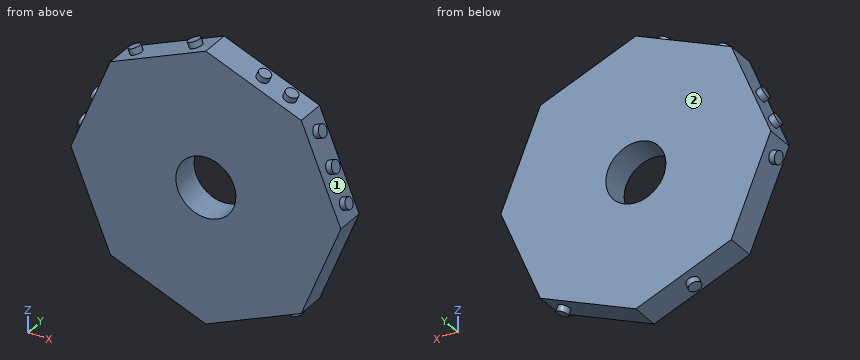
from build123d import *

# Parameters (mm, degrees)
BOSS_EXTRUDE1_DEPTH      = 12.7
SKETCH6_R                = 2.582336278
BOSS_EXTRUDE5_DEPTH      = 2.54
SKETCH8_R                = 2.650649738
BOSS_EXTRUDE7_DEPTH      = 2.54
SKETCH9_R                = 2.655151376
BOSS_EXTRUDE8_DEPTH      = 2.54
BOSS_EXTRUDE9_DEPTH      = 2.54
BOSS_EXTRUDE9_DEPTH_BACK = 2.032
SKETCH10_R               = 2.513561162
SKETCH11_R               = 2.58621177
BOSS_EXTRUDE10_DEPTH     = 2.54
SKETCH12_R               = 2.635427952
BOSS_EXTRUDE11_DEPTH     = 2.54
SKETCH13_R               = 2.610060734
BOSS_EXTRUDE12_DEPTH     = 2.54
SKETCH14_R               = 2.635257061
BOSS_EXTRUDE13_DEPTH     = 2.54
SKETCH15_R               = 2.496375984
BOSS_EXTRUDE14_DEPTH     = 2.54
SKETCH16_R               = 2.621965254
BOSS_EXTRUDE15_DEPTH     = 2.54
SKETCH17_R               = 2.649584499
BOSS_EXTRUDE16_DEPTH     = 2.54
SKETCH18_R               = 2.417668351
BOSS_EXTRUDE17_DEPTH     = 2.54
SKETCH25_R               = 12.696845274
CUT_EXTRUDE1_DEPTH       = 12.954


with BuildPart() as part:
    # Sketch2 → Boss-Extrude1 (new body)
    with BuildSketch(Plane(origin=(0, 0, 0), x_dir=(1, 0, 0), z_dir=(0, 1, 0))):
        Polygon((57.113851186, 0), (40.385591473, 40.385591473), (0, 57.113851186), (-40.385591473, 40.385591473), (-57.113851186, 0), (-40.385591473, -40.385591473), (0, -57.113851186), (40.385591473, -40.385591473), align=None)
    extrude(amount=BOSS_EXTRUDE1_DEPTH)

    # Sketch6 → Boss-Extrude5 (add)
    with BuildSketch(Plane(origin=(20.192795737, 0, 48.749721329), x_dir=(0.9238795325112822, 0, -0.38268343236510083), z_dir=(0.38268343236510083, 0, 0.9238795325112822))):
        with Locations(Location((0, 6.35, 0), (0, 0, 180))):
            Circle(SKETCH6_R)
    extrude(amount=BOSS_EXTRUDE5_DEPTH)

    # Sketch8 → Boss-Extrude7 (add)
    with BuildSketch(Plane(origin=(20.192795737, 0, 48.749721329), x_dir=(0.9238795325112822, 0, -0.38268343236510083), z_dir=(0.38268343236510083, 0, 0.9238795325112822))):
        with Locations(Location((12.369517224, 6.35, 0), (0, 0, 180))):
            Circle(SKETCH8_R)
    extrude(amount=BOSS_EXTRUDE7_DEPTH)

    # Sketch9 → Boss-Extrude8 (add)
    with BuildSketch(Plane(origin=(-20.192795737, 0, 48.749721329), x_dir=(0.9238795325112911, 0, 0.38268343236507935), z_dir=(-0.38268343236507935, 0, 0.9238795325112911))):
        with Locations(Location((13.282722146, 6.35, 0), (0, 0, 180))):
            Circle(SKETCH9_R)
    extrude(amount=BOSS_EXTRUDE8_DEPTH)

    # Sketch10 → Boss-Extrude9 (add, two sides: drawn at the far end of the back side and taken through both)
    with BuildSketch(Plane(origin=(-20.192795737, 0, 48.749721329), x_dir=(0.9238795325112911, 0, 0.38268343236507935), z_dir=(-0.38268343236507935, 0, 0.9238795325112911)).offset(-BOSS_EXTRUDE9_DEPTH_BACK)):
        with Locations(Location((-14.008863044, 6.35, 0), (0, 0, 180))):
            Circle(SKETCH10_R)
    extrude(amount=BOSS_EXTRUDE9_DEPTH + BOSS_EXTRUDE9_DEPTH_BACK)

    # Sketch11 → Boss-Extrude10 (add)
    with BuildSketch(Plane(origin=(-48.749721329, 0, 20.192795737), x_dir=(0.3826834323651003, 0, 0.9238795325112825), z_dir=(-0.9238795325112825, 0, 0.3826834323651003))):
        with Locations(Location((-13.637069306, 6.35, 0), (0, 0, 180))):
            Circle(SKETCH11_R)
    extrude(amount=BOSS_EXTRUDE10_DEPTH)

    # Sketch12 → Boss-Extrude11 (add)
    with BuildSketch(Plane(origin=(-48.749721329, 0, 20.192795737), x_dir=(0.3826834323651003, 0, 0.9238795325112825), z_dir=(-0.9238795325112825, 0, 0.3826834323651003))):
        with Locations(Location((0, 6.35, 0), (0, 0, 180))):
            Circle(SKETCH12_R)
    extrude(amount=BOSS_EXTRUDE11_DEPTH)

    # Sketch13 → Boss-Extrude12 (add)
    with BuildSketch(Plane(origin=(-48.749721329, 0, -20.192795737), x_dir=(-0.38268343236507907, 0, 0.9238795325112913), z_dir=(-0.9238795325112913, 0, -0.38268343236507907))):
        with Locations(Location((14.354264816, 6.35, 0), (0, 0, 180))):
            Circle(SKETCH13_R)
    extrude(amount=BOSS_EXTRUDE12_DEPTH)

    # Sketch14 → Boss-Extrude13 (add)
    with BuildSketch(Plane(origin=(-20.192795737, 0, -48.749721329), x_dir=(-0.9238795325112825, 0, 0.3826834323651002), z_dir=(-0.3826834323651002, 0, -0.9238795325112825))):
        with Locations(Location((0, 6.35, 0), (0, 0, 180))):
            Circle(SKETCH14_R)
    extrude(amount=BOSS_EXTRUDE13_DEPTH)

    # Sketch15 → Boss-Extrude14 (add)
    with BuildSketch(Plane(origin=(20.192795737, 0, -48.749721329), x_dir=(-0.9238795325112913, 0, -0.38268343236507896), z_dir=(0.3826834323650789, 0, -0.9238795325112912))):
        with Locations(Location((-15.021400656, 6.35, 0), (0, 0, 180))):
            Circle(SKETCH15_R)
    extrude(amount=BOSS_EXTRUDE14_DEPTH)

    # Sketch16 → Boss-Extrude15 (add)
    with BuildSketch(Plane(origin=(48.749721329, 0, 20.192795737), x_dir=(0.3826834323650791, 0, -0.9238795325112912), z_dir=(0.9238795325112913, 0, 0.3826834323650792))):
        with Locations(Location((-14.377366693, 6.35, 0), (0, 0, 180))):
            Circle(SKETCH16_R)
    extrude(amount=BOSS_EXTRUDE15_DEPTH)

    # Sketch17 → Boss-Extrude16 (add)
    with BuildSketch(Plane(origin=(48.749721329, 0, 20.192795737), x_dir=(0.3826834323650791, 0, -0.9238795325112912), z_dir=(0.9238795325112913, 0, 0.3826834323650792))):
        with Locations(Location((0, 6.35, 0), (0, 0, 180))):
            Circle(SKETCH17_R)
    extrude(amount=BOSS_EXTRUDE16_DEPTH)

    # Sketch18 → Boss-Extrude17 (add)
    with BuildSketch(Plane(origin=(48.749721329, 0, 20.192795737), x_dir=(0.3826834323650791, 0, -0.9238795325112912), z_dir=(0.9238795325112913, 0, 0.3826834323650792))):
        with Locations(Location((14.696818613, 6.35, 0), (0, 0, 180))):
            Circle(SKETCH18_R)
    extrude(amount=BOSS_EXTRUDE17_DEPTH)

    # Sketch25 → Cut-Extrude1 (cut)
    with BuildSketch(Plane(origin=(0, 12.7, 0), x_dir=(1, 0, 0), z_dir=(0, 1, 0))):
        with Locations(Location((0, 0, 0), (0, 0, 270))):
            Circle(SKETCH25_R)
    extrude(amount=-CUT_EXTRUDE1_DEPTH, mode=Mode.SUBTRACT)


solid = part.part
CAD build for the part. Positions are in the model's coordinates, mm. Face numbers are marked on the shaded views. Round coordinates to 2 decimals unless told otherwise and drop trailing zeros. Order: outer loops, then holes, each group sorted by start corner. A loop starts at its lowest first (then second) coordinate and runs counter-clockwise, first axis right, second up. Notation, with made-up numbers: (62.5, 88.5) - (88.5, 88.5) arc R19 cw to (88.5, 111.5) - close; hole circle Ø6 at (-9.75, -7). An arc over 180 degrees is marked (long way). Return JSON: item names as keys, results as strings.
(1) Cut at B-B (z = 1.5). Give the cut face in (x, y).
Answer key:
{"outline": "(-56.49, 0) - (-12.61, 0) - (-12.61, 12.7) - (-56.49, 12.7) - close; (12.61, 0) - (56.49, 0) - (56.49, 12.7) - (12.61, 12.7) - close"}
(2) Pin check, flat tips, straight feed: pin 1 Ø1 at (x, y) = (43.5, 5.5) entering from +Z; pin 2 Ø6 at (x, y) = (-14.5, 9) entering from -Z; pin 3 Ø10 at (x, z) = (7, -13) entering from -Y; pin 4 Ø2 at (y, z) = (11, -26) entering from -X. Stop position of each tip, or through.
Answer key:
{"pin 1": "stops at z = 36.52", "pin 2": "stops at z = -52.35", "pin 3": "stops at y = 0", "pin 4": "stops at x = -46.76"}
(3) Cut at A-A (y = 11). Give the cut face in (x, z), then the cut area to 3 significant figures.
Answer key:
{"outline": "(-57.11, 0) - (-40.39, -40.39) - (0, -57.11) - (40.39, -40.39) - (57.11, 0) - (40.39, 40.39) - (0, 57.11) - (-40.39, 40.39) - close; hole circle Ø25.39 at (0, 0)", "area": "8,720 mm^2"}
(4) Wall check: probe 1 along X at (y, z) = (7.25, 0); probe 2 along X at (y, z) = (5.75, -3.5); probe 3 along Z at (x, y) = (10, 6). Give the ranges that are in metal, low to high. Write a range as from..to.
Answer key:
{"probe 1": "x = -57.11..-12.7, 12.7..57.11", "probe 2": "x = -55.66..-12.2, 12.2..55.66", "probe 3": "z = -52.97..-7.82, 7.82..52.97"}
(5) Pull direction Z, two halves, no side cores. Call the marked faces 1 and 2: +Z half, -Z half, draft (parallel to the pull), parting line (faces both ways), or undercut.
Answer key:
{"face 1": "undercut", "face 2": "draft"}
(6) Cut at D-D (z = 14.5). Give the cut face in (x, y).
Answer key:
{"outline": "(-51.11, 0) - (51.11, 0) - (51.11, 12.7) - (-51.11, 12.7) - close"}
(7) Cut at C-C (x = -15). Give the cut face in (y, z), then the cut area to 3 significant figures.
Answer key:
{"outline": "(0, -50.9) - (12.7, -50.9) - (12.7, 50.9) - (0, 50.9) - close", "area": "1,290 mm^2"}
